```python
from build123d import *

# Parameters (mm, degrees)
F1_DEPTH      = 7.9375
F1_DEPTH_BACK = 7.9375
F2_R          = 6.35
F3_R          = 3.302
F4_DEPTH      = 25.4
F6_DEPTH      = 4.7625
F7_R          = 2.54
F9_DEPTH      = 4.7625
F10_R         = 4.826
F11_DEPTH     = 38.101


with BuildPart() as f1:
    # F0 (on Front) → F1 (new body, two sides)
    with BuildSketch(Plane.XZ) as f1_sk:
        Polygon((0, 19.05), (0, 0), (25.4, 0), (38.1, -19.05), (50.8, -19.05), (50.8, 19.05), align=None)
    extrude(amount=F1_DEPTH)
    extrude(f1_sk.sketch, amount=-F1_DEPTH_BACK)

    # F2
    f2_edges = [f1.edges().sort_by_distance(p)[0] for p in [
        (25.4, 0, 0),
        (38.1, 0, -19.05),
        (50.8, 0, -19.05),
    ]]
    fillet(f2_edges, radius=F2_R)

    # F3 (on face) → F4 (cut)
    with BuildSketch(Plane.XZ.offset(7.9375)):
        with Locations((42.974208, -12.7)):
            Circle(F3_R)
        with Locations((42.974208, 12.7)):
            Circle(F3_R)
    extrude(amount=-F4_DEPTH, mode=Mode.SUBTRACT)

    # F5 (on face) → F6 (cut)
    with BuildSketch(Plane.XZ.offset(7.9375)):
        with BuildLine():
            Line((42.974208, -12.7), (42.974208, 1.5875))
            ThreePointArc((42.974208, 1.5875), (32.87142, -22.802788), (57.261708, -12.7))
            Line((57.261708, -12.7), (42.974208, -12.7))
        make_face()
        with BuildLine():
            ThreePointArc((54.086708, 12.7), (35.116484, 20.557724), (42.974208, 1.5875))
            Line((42.974208, 1.5875), (42.974208, 12.7))
            Line((42.974208, 12.7), (54.086708, 12.7))
        make_face()
        Polygon((42.974208, 12.7), (42.974208, 1.5875), (42.974208, -12.7), (57.261708, -12.7), (61.707854, -12.7), (61.707854, 12.7), (54.086708, 12.7), align=None)
    extrude(amount=-F6_DEPTH, mode=Mode.SUBTRACT)

    # F7
    f7_edges = [f1.edges().sort_by_distance(p)[0] for p in [
        (42.974208, -5.55625, 1.5875),
    ]]
    fillet(f7_edges, radius=F7_R)

    # F8 (on face) → F9 (cut)
    with BuildSketch(Plane(origin=(0, 7.9375, 0), x_dir=(-1, 0, 0), z_dir=(0, 1, 0))):
        with BuildLine():
            Line((-50.8, 19.05), (-50.8, -12.7))
            ThreePointArc((-50.8, -12.7), (-48.940128, -17.190128), (-44.45, -19.05))
            Line((-44.45, -19.05), (-41.498417, -19.05))
            ThreePointArc((-41.498417, -19.05), (-38.502119, -18.298634), (-36.214897, -16.222346))
            Line((-36.214897, -16.222346), (-29.950297, -6.825446))
            ThreePointArc((-29.950297, -6.825446), (-32.398052, -3.093879), (-35.877663, -0.299528))
            ThreePointArc((-35.877663, -0.299528), (-37.149918, 1.728535), (-36.17106, 3.913372))
            ThreePointArc((-36.17106, 3.913372), (-31.989583, 11.019032), (-33.854715, 19.05))
            Line((-33.854715, 19.05), (-50.8, 19.05))
        make_face()
    extrude(amount=-F9_DEPTH, mode=Mode.SUBTRACT)

    # F10 (on face) → F11 (cut, through all)
    with BuildSketch(Plane.XY.offset(19.05)):
        with Locations((12.7, 0)):
            Circle(F10_R)
    extrude(amount=-F11_DEPTH, mode=Mode.SUBTRACT)


solid = f1.part
```
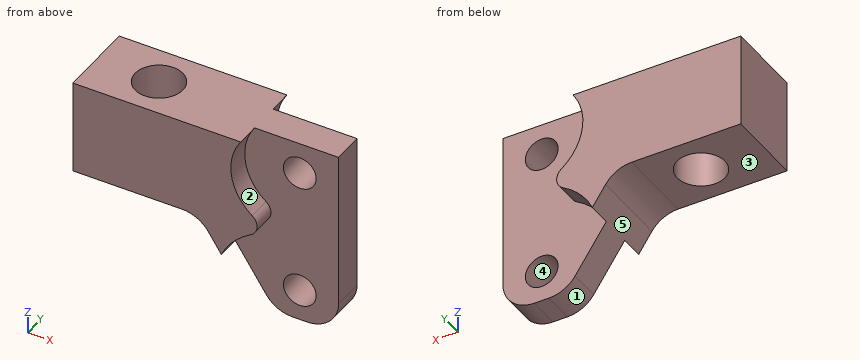
Verification items for the finished model (mm, model axes). Face numbers are marked on the shaded views. A direction names the side the tool comes from. Round coordinates to 2 decimals unless told otherwise and drop trailing zeros. Write each loop counter-clockwise with the first axis right and the second up, starting at its lowest first coordinate (ties: lowest second). Pieces come first, ordered by that corner, then holes. Notation, with made-up numbers: (24, 14) - (51, 14) arc R26 ccw to (51, 45) - close; hole circle Ø2 at (57, 64.5). An arc over 180 degrees is marked (long way). Answer as a JSON object with one key per item and string values. Group by question number.
Q1. Section check C-C, the plane x = 12.7. Enter the section's corners in (y, z).
Q2. Section check D-D, the plane z = -11. Enter the section's corners in (x, y) (3 decimals).
Q3. Section check A-A, the plane z = 12.7. Enter the section's corners in (x, y) (1 decimal).
Q4. Mould release check, pull along X, two halves, no side actions. Record for the marked faces 3, 4 and 5: released by +X, released by -X, zero draft, split by the parting line, or undercut.
Q5. Section check B-B, the plane y = -1.25. Enter the section's corners in (x, z), plus the area to 3 significant figures.
Q6. Thickness scan on line 1 (Y direction, x = 34.5, z = 6.5) (3 decimals); line 2 (Y direction, x = 12.7, z = 8.75); line 3 (Z direction, x = 33.5, y = 4). Record the ranges inside material, lowest first.
Q7. Go/stop test with flat-tipped pins: pin 1 Ø1.5 at (x, z) = (43.5, 13) entering from -Y; pin 2 Ø16.5 at (x, z) = (44, -6.5) entering from -Y (3 decimals); pin 3 Ø1 at (x, y) = (20.5, 3.5) entering from -Z; pin 4 Ø1 at (x, z) = (39.5, 11.5) entering from +Y (3 decimals). Record where each tip stops, or that it passes through.
Q8. Tool access check on the marked faces 1 and 2. Record the directions out of +Z, -Z, +X, -X, +Y, -Y that give a thin tool (end or side, any length) a straight path to the whole face; none if there is none.
Found:
{
 "1": {"outline": "(-7.94, 0) - (-4.83, 0) - (-4.83, 19.05) - (-7.94, 19.05) - close; (4.83, 0) - (7.94, 0) - (7.94, 19.05) - (4.83, 19.05) - close"},
 "2": {"outline": "(32.733, -3.175) - (40.143, -3.175) - (40.143, 3.175) - (32.733, 3.175) - close; (45.805, -3.175) - (50.8, -3.175) - (50.8, 3.175) - (45.805, 3.175) - close"},
 "3": {"outline": "(0, -7.9) - (31.9, -7.9) - (31.9, -3.2) - (39.7, -3.2) - (39.7, 3.2) - (31.9, 3.2) - (31.9, 7.9) - (0, 7.9) - close; (46.3, -3.2) - (50.8, -3.2) - (50.8, 3.2) - (46.3, 3.2) - close; hole circle Ø9.7 at (12.7, 0)"},
 "4": {"face 3": "zero draft", "face 4": "undercut", "face 5": "released by -X"},
 "5": {"outline": "(0, 0) - (8.04, 0) - (8.04, 19.05) - (0, 19.05) - close; (17.36, 0) - (22, 0) arc R6.35 cw to (27.29, -2.83) - (36.21, -16.22) arc R6.35 ccw to (41.5, -19.05) - (44.45, -19.05) arc R6.35 ccw to (50.8, -12.7) - (50.8, 19.05) - (17.36, 19.05) - close; hole circle Ø6.6 at (42.97, -12.7); hole circle Ø6.6 at (42.97, 12.7)", "area": "1,080 mm^2"},
 "6": {"line 1": "y = -3.175 to 3.175", "line 2": "y = -7.94 to -4.83, 4.83 to 7.94", "line 3": "z = -2.01 to 6.89, 18.51 to 19.05"},
 "7": {"pin 1": "passes through", "pin 2": "stops at y = -3.175", "pin 3": "stops at z = 0", "pin 4": "stops at y = 3.175"},
 "8": {"face 1": "-Z, -X, +Y, -Y", "face 2": "+X, -Y"}
}
